Part model, mm, in its own coordinate system. A direction names the side the tool comes from. Round coordinates to 2 decimals unless told otherwise and drop trailing zeros. Loops run counter-clockwise (first coordinate to the right, second up) from the corner with the lowest first, then second, coordinate; pieces in that order, holes last. Notation, with made-up numbers: (29.25, -35) -> (42.25, -35) arc R12 ccw to (42.25, -23) -> close; hole circle Ø3 at (45, 68). An arc over 180 degrees is marked (long way). Answer as a JSON object with one key per item and string values. Group by question number.
from build123d import *

# Parameters (mm, degrees)
BOSS_EXTRUDE1_DEPTH = 15
SKETCH2_R           = 7.5
CUT_EXTRUDE1_DEPTH  = 15
BOSS_EXTRUDE2_DEPTH = 50
SKETCH4_R           = 12.5
CUT_EXTRUDE2_DEPTH  = 50
BOSS_EXTRUDE3_DEPTH = 5


with BuildPart() as part:
    # Sketch1 → Boss-Extrude1 (new body)
    with BuildSketch(Plane(origin=(0, 0, 0), x_dir=(1, 0, 0), z_dir=(0, 1, 0))):
        with BuildLine():
            Line((85, -50), (-85, -50))
            ThreePointArc((-85, -50), (-95.606601718, -45.606601718), (-100, -35))
            Line((-100, -35), (-100, 35))
            ThreePointArc((-100, 35), (-95.606601718, 45.606601718), (-85, 50))
            Line((-85, 50), (85, 50))
            ThreePointArc((85, 50), (95.606601718, 45.606601718), (100, 35))
            Line((100, 35), (100, -35))
            ThreePointArc((100, -35), (95.606601718, -45.606601718), (85, -50))
        make_face()
    extrude(amount=BOSS_EXTRUDE1_DEPTH)

    # Sketch2 → Cut-Extrude1 (cut)
    with BuildSketch(Plane(origin=(0, 15, 0), x_dir=(1, 0, 0), z_dir=(0, 1, 0))):
        with Locations((-85, 35)):
            Circle(SKETCH2_R)
        with Locations((-85, -35)):
            Circle(SKETCH2_R)
        with Locations((85, -35)):
            Circle(SKETCH2_R)
        with Locations((85, 35)):
            Circle(SKETCH2_R)
    extrude(amount=-CUT_EXTRUDE1_DEPTH, mode=Mode.SUBTRACT)

    # Sketch3 → Boss-Extrude2 (add, symmetric)
    with BuildSketch(Plane.XY):
        with BuildLine():
            Line((-45.424155313, 15), (-21.336304632, 91.970721254))
            ThreePointArc((-21.336304632, 91.970721254), (0, 130), (21.336304632, 91.970721254))
            Line((21.336304632, 91.970721254), (45.424155313, 15))
            Line((45.424155313, 15), (-45.424155313, 15))
        make_face()
    extrude(amount=BOSS_EXTRUDE2_DEPTH, both=True)

    # Sketch4 → Cut-Extrude2 (cut, symmetric)
    with BuildSketch(Plane.XY):
        with Locations((0, 105)):
            Circle(SKETCH4_R)
    extrude(amount=CUT_EXTRUDE2_DEPTH, both=True, mode=Mode.SUBTRACT)

    # Sketch6 → Boss-Extrude3 (add, symmetric)
    with BuildSketch(Plane.XY):
        Polygon((-85.424155313, 15), (-27.204379859, 73.219775454), (-45.424155313, 15), align=None)
        Polygon((45.424155313, 15), (27.204379859, 73.219775454), (85.424155313, 15), align=None)
    extrude(amount=BOSS_EXTRUDE3_DEPTH, both=True)


solid = part.part
Item 1: Drop flat-ended pins along their axis: pin 1 Ø24 at (x, z) = (85, -35) entering from +Y; pin 2 Ø24 at (x, z) = (-85, -35) entering from -Y; pin 3 Ø5 at (y, z) = (56, 27) entering from +X; pin 4 Ø2 at (y, z) = (26.5, -13.5) entering from -X. Give the stop position or say it passes through.
Item 2: Band-saw the part on B-B, the plane y = 11. List the corners of the cut face in (x, z).
Item 3: Band-saw the part on D-D, the plane z = 17. List the corners of the cut face in (x, y), plus the area to 3 significant figures.
Item 4: Drill centre lines: line 1 (Z direction, x = -85, y = 7); line 2 (X direction, y = 10, z = 35); line 3 (Y direction, x = 92, z = -42). Where is each one in solid material? Low to high.
Item 5: Band-saw the part on C-C, the plane y = 105. List the corners of the cut face in (x, z).
Item 6: Which spindle directions (+Z, -Z, +X, -X, +Y, -Y) get a long thin tool onto all of the face, cutting with end or side? Do faces 1 (the face through (33.212, 54.024, 11.811)), 2 (the face through (-72, 15, 10)), 3 (the face through (73, 15, -12)). Say none if no direction does.
Item 7: Two-plate mould, pull along Z, no slides. Class faces 4 (the face through (79.048, 7.605, -30.436)), 5 (the face through (-33.549, 52.947, 11.811)), 6 (the face through (-90.952, 7.605, -30.436)), 7 (the face through (-52, 33, 5)): pulls with the +Z half, pulls with the -Z half, needs draft (parallel to the pull), parting line crosses it, or undercut.
Item 8: Band-saw the part on A-A, the plane x = 0. List the corners of the cut face in (y, z).
Entries:
{
 "1": {"pin 1": "y = 15", "pin 2": "y = 0", "pin 3": "x = 33.38", "pin 4": "x = -42.14"},
 "2": {"outline": "(-100, -35) arc R15 ccw to (-85, -50) -> (85, -50) arc R15 ccw to (100, -35) -> (100, 35) arc R15 ccw to (85, 50) -> (-85, 50) arc R15 ccw to (-100, 35) -> close; hole circle Ø15 at (-85, -35); hole circle Ø15 at (-85, 35); hole circle Ø15 at (85, -35); hole circle Ø15 at (85, 35)"},
 "3": {"outline": "(-100, 0) -> (100, 0) -> (100, 15) -> (45.42, 15) -> (21.34, 91.97) arc R25 ccw (long way) to (-21.34, 91.97) -> (-45.42, 15) -> (-100, 15) -> close; hole circle Ø25 at (0, 105)", "area": "9,250 mm²"},
 "4": {"line 1": "-50 to -42.5, -27.5 to 27.5, 42.5 to 50", "line 2": "-100 to -92.5, -77.5 to 77.5, 92.5 to 100", "line 3": "0 to 15"},
 "5": {"outline": "(-25, -50) -> (-12.5, -50) -> (-12.5, 50) -> (-25, 50) -> close; (12.5, -50) -> (25, -50) -> (25, 50) -> (12.5, 50) -> close"},
 "6": {"face 1": "+X", "face 2": "-X, +Y", "face 3": "+X, +Y"},
 "7": {"face 4": "undercut", "face 5": "needs draft", "face 6": "undercut", "face 7": "pulls with the +Z half"},
 "8": {"outline": "(0, -50) -> (92.5, -50) -> (92.5, 50) -> (0, 50) -> close; (117.5, -50) -> (130, -50) -> (130, 50) -> (117.5, 50) -> close"}
}
